from build123d import *

# Parameters (mm, degrees)
BOSS_EXTRUDE1_DEPTH = 30
SKETCH4_W           = 30
SKETCH4_H           = 11.480502971
BOSS_EXTRUDE2_DEPTH = 50
CUT_EXTRUDE1_DEPTH  = 5
CUT_EXTRUDE3_DEPTH  = 6.480502971
FILLET1_R           = 10
CHAMFER3_SIZE       = 22.5
CHAMFER3_SIZE2      = 8.610377228
CHAMFER1_SIZE       = 15
CHAMFER1_SIZE2      = 20.645728807
CHAMFER2_SIZE2      = 20.645728807
CHAMFER2_SIZE       = 15
CUT_EXTRUDE4_DEPTH  = 25
CUT_EXTRUDE5_DEPTH  = 25
SKETCH9_W           = 20.645728807
SKETCH9_H           = 30
CUT_EXTRUDE6_DEPTH  = 40
SKETCH10_W          = 10
SKETCH10_H          = 12.413129657
BOSS_EXTRUDE3_DEPTH = 12
SKETCH11_W          = 31
SKETCH11_H          = 30
CUT_EXTRUDE7_DEPTH  = 2
SKETCH12_W          = 25.5
SKETCH12_H          = 20
CUT_EXTRUDE8_DEPTH  = 4
CHAMFER4_SIZE       = 2
CUT_EXTRUDE9_DEPTH  = 30
SKETCH16_W          = 6
SKETCH16_H          = 20
CUT_EXTRUDE10_DEPTH = 30.1
CHAMFER6_SIZE       = 2
BOSS_EXTRUDE4_DEPTH = 25.5
SKETCH18_W          = 2.6
SKETCH18_H          = 4.5
BOSS_EXTRUDE5_DEPTH = 10
CHAMFER7_SIZE       = 1
FILLET2_R           = 5
CHAMFER8_SIZE       = 8


with BuildPart() as part:
    # Sketch1 → Boss-Extrude1 (new body)
    with BuildSketch(Plane.XY):
        Polygon((0, 216.478440058), (-153.073372946, 153.073372946), (-216.478440058, 0), (-244.194826034, 0), (-244.194826034, 11.480502971), (-176.034378888, 176.034378888), (0, 248.950206067), align=None)
    extrude(amount=BOSS_EXTRUDE1_DEPTH)

    # Sketch4 → Boss-Extrude2 (add)
    with BuildSketch(Plane.ZY.offset(244.194826034)):
        with Locations((15, 5.740251485)):
            Rectangle(SKETCH4_W, SKETCH4_H)
    extrude(amount=BOSS_EXTRUDE2_DEPTH)

    # Sketch5 → Cut-Extrude1 (cut)
    with BuildSketch(Plane(origin=(0, 11.480502971, 0), x_dir=(1, 0, 0), z_dir=(0, 1, 0))):
        with BuildLine():
            Line((-281.694826034, -6), (-256.694826034, -6))
            ThreePointArc((-256.694826034, -6), (-247.694826034, -15), (-256.694826034, -24))
            Line((-256.694826034, -24), (-281.694826034, -24))
            ThreePointArc((-281.694826034, -24), (-290.694826034, -15), (-281.694826034, -6))
        make_face()
    extrude(amount=-CUT_EXTRUDE1_DEPTH, mode=Mode.SUBTRACT)

    # Sketch7 → Cut-Extrude3 (cut)
    with BuildSketch(Plane(origin=(0, 6.480502971, 0), x_dir=(1, 0, 0), z_dir=(0, 1, 0))):
        with BuildLine():
            Line((-256.694826034, -11.5), (-281.694826034, -11.5))
            ThreePointArc((-281.694826034, -11.5), (-285.194826034, -15), (-281.694826034, -18.5))
            Line((-281.694826034, -18.5), (-256.694826034, -18.5))
            ThreePointArc((-256.694826034, -18.5), (-253.194826034, -15), (-256.694826034, -11.5))
        make_face()
    extrude(amount=-CUT_EXTRUDE3_DEPTH, mode=Mode.SUBTRACT)

    # Fillet1
    fillet1_edges = [part.edges().sort_by_distance(p)[0] for p in [
        (-294.194826034, 5.740251485, 0),
        (-294.194826034, 5.740251485, 30),
    ]]
    fillet(fillet1_edges, radius=FILLET1_R)

    # Chamfer3
    chamfer3_edges = [part.edges().sort_by_distance(p)[0] for p in [
        (0, 248.950206067, 15),
    ]]
    chamfer3_side = [part.faces().sort_by_distance(p)[0] for p in [
        (-88.017189444, 212.492292478, 15),
    ]]
    chamfer(chamfer3_edges, length=CHAMFER3_SIZE, length2=CHAMFER3_SIZE2, reference=chamfer3_side[0])

    # Chamfer1
    chamfer1_edges = [part.edges().sort_by_distance(p)[0] for p in [
        (0, 228.409134449, 0),
    ]]
    chamfer1_side = [part.faces().sort_by_distance(p)[0] for p in [
        (0, 228.409134449, 15),
    ]]
    chamfer(chamfer1_edges, length=CHAMFER1_SIZE, length2=CHAMFER1_SIZE2, reference=chamfer1_side[0])

    # Chamfer2
    chamfer2_edges = [part.edges().sort_by_distance(p)[0] for p in [
        (0, 228.409134449, 30),
    ]]
    chamfer2_side = [part.faces().sort_by_distance(p)[0] for p in [
        (0, 228.409134449, 29.7),
    ]]
    chamfer(chamfer2_edges, length=CHAMFER2_SIZE - 0.0001, length2=CHAMFER2_SIZE2 - 0.0001, reference=chamfer2_side[0])  # a hair under: the kernel refuses the full size

    # Sketch3 → Cut-Extrude4 (cut)
    with BuildSketch(Plane.XY.offset(30)):
        Polygon((-186.689323664, 71.91728881), (-182.86248934, 81.156084136), (-192.101284666, 84.982918459), (-184.129988769, 104.227329121), (-202.60757942, 111.880997769), (-206.434413743, 102.642202444), (-194.423979821, 97.667317823), (-203.608382197, 75.494209043), (-197.14122547, 72.815425016), (-195.928118989, 75.744123134), align=None)
        Polygon((-81.156084136, 182.86248934), (-71.91728881, 186.689323664), (-75.744123134, 195.928118989), (-72.815425016, 197.14122547), (-75.494209043, 203.608382197), (-97.667317823, 194.423979821), (-102.642202444, 206.434413743), (-111.880997769, 202.60757942), (-106.906113148, 190.597145497), (-104.227329121, 184.129988769), (-84.982918459, 192.101284666), align=None)
    extrude(amount=-CUT_EXTRUDE4_DEPTH, mode=Mode.SUBTRACT)

    # Sketch8 → Cut-Extrude5 (cut)
    with BuildSketch(Plane.XY.offset(30)):
        Polygon((-66.282610192, 194.435244969), (-67.813343921, 198.130763099), (-66.889464389, 198.513446531), (-70.716298712, 207.752241857), (-71.640178245, 207.369558424), (-73.170911974, 211.065076554), (-72.247032442, 211.447759987), (-74.925816468, 217.914916714), (-46.28555096, 229.778103118), (-43.606766934, 223.31094639), (-38.987369271, 225.224363552), (-37.456635542, 221.528845422), (-42.076033204, 219.61542826), (-38.249198881, 210.376632935), (-33.629801218, 212.290050097), (-32.099067489, 208.594531967), align=None)
    extrude(amount=-CUT_EXTRUDE5_DEPTH, mode=Mode.SUBTRACT)

    # Sketch9 → Cut-Extrude6 (cut)
    with BuildSketch(Plane(origin=(0, 240.339828839, 0), x_dir=(1, 0, 0), z_dir=(0, 1, 0))):
        with Locations((-10.322864404, -15)):
            Rectangle(SKETCH9_W, SKETCH9_H)
    extrude(amount=-CUT_EXTRUDE6_DEPTH, mode=Mode.SUBTRACT)


with BuildPart() as cut_extrude6_kept_piece:
    # of the separate pieces the step leaves, the one the design keeps (cut_extrude6_pieces_kept)
    add(part.part.solids().sort_by_distance((-20.787289482, 240.339828839, 30))[0])

    # Sketch10 → Boss-Extrude3 (add)
    with BuildSketch(Plane(origin=(-20.645728807, 0, 0), x_dir=(0, 0, -1), z_dir=(1, 0, 0))):
        with Locations((-15, 224.13326401)):
            Rectangle(SKETCH10_W, SKETCH10_H)
    extrude(amount=BOSS_EXTRUDE3_DEPTH)

    # Sketch11 → Cut-Extrude7 (cut)
    with BuildSketch(Plane(origin=(-76.536686473, 184.775906502, 0), x_dir=(0.9238795325112865, 0.38268343236509045, 0), z_dir=(0.38268343236509045, -0.9238795325112865, 0))):
        with Locations((0.5, 15)):
            Rectangle(SKETCH11_W, SKETCH11_H)
    extrude(amount=-CUT_EXTRUDE7_DEPTH, mode=Mode.SUBTRACT)

    # Sketch12 → Cut-Extrude8 (cut)
    with BuildSketch(Plane(origin=(-184.775906502, 76.536686473, 0), x_dir=(0, 0, -1), z_dir=(0.9238795325112872, -0.38268343236508917, 0))):
        with Locations((-17.25, 0)):
            Rectangle(SKETCH12_W, SKETCH12_H)
    extrude(amount=-CUT_EXTRUDE8_DEPTH, mode=Mode.SUBTRACT)

    # Chamfer4
    chamfer4_edges = [cut_extrude6_kept_piece.edges().sort_by_distance(p)[0] for p in [
        (-111.880997769, 202.60757942, 17.5),
        (-102.642202444, 206.434413743, 17.5),
        (-83.45218473, 188.405766535, 30),
        (-74.279774075, 196.534672229, 30),
        (-74.154817029, 200.374803834, 30),
        (-86.580763433, 199.016181009, 30),
        (-100.154760133, 200.429196782, 30),
        (-108.054163445, 193.368784094, 30),
        (-94.60512379, 188.115636717, 30),
        (-206.434413743, 102.642202444, 17.5),
        (-188.115636717, 94.60512379, 30),
        (-193.368784094, 108.054163445, 30),
        (-200.429196782, 100.154760133, 30),
        (-199.016181009, 86.580763433, 30),
        (-200.374803834, 74.154817029, 30),
        (-196.534672229, 74.279774075, 30),
        (-193.156480392, 74.596072837, 30),
        (-49.19083884, 201.514888468, 30),
        (-32.864434353, 210.442291032, 30),
        (-40.162616043, 214.996030597, 30),
        (-38.222002407, 223.376604487, 30),
        (-72.40554511, 209.217317489, 30),
        (-67.047977056, 196.283004034, 30),
        (-74.213389405, 192.232600859, 30),
        (-81.921451, 184.710248405, 17.5),
        (-72.682655675, 188.537082729, 17.5),
        (-189.329646068, 83.834868162, 30),
        (-186.55800747, 82.686817865, 17.5),
        (-190.384841794, 73.44802254, 17.5),
    ]]
    chamfer(chamfer4_edges, length=CHAMFER4_SIZE)

    # Sketch13 → Cut-Extrude9 (cut)
    with BuildSketch(Plane(origin=(0, 0, 0), x_dir=(-1, 0, 0), z_dir=(0, 0, -1))):
        Polygon((180.789758921, 164.553875917), (153.073372946, 153.073372946), (-25.433862624, 226.424491684), (-10.416597064, 262.970499532), (187.527299345, 181.632585119), align=None)
    extrude(amount=-CUT_EXTRUDE9_DEPTH, mode=Mode.SUBTRACT)

    # Sketch16 → Cut-Extrude10 (cut)
    with BuildSketch(Plane(origin=(31.702533556, 76.536686473, 0), x_dir=(0.9238795325112868, -0.38268343236508956, 0), z_dir=(0.38268343236508956, 0.9238795325112868, 0))):
        with Locations((-227, -15)):
            Rectangle(SKETCH16_W, SKETCH16_H)
        with Locations((-203, -15)):
            Rectangle(SKETCH16_W, SKETCH16_H)
    extrude(amount=-CUT_EXTRUDE10_DEPTH, mode=Mode.SUBTRACT)

    # Chamfer6
    chamfer6_edges = [cut_extrude6_kept_piece.edges().sort_by_distance(p)[0] for p in [
        (-178.018120324, 163.40582562, 25),
        (-175.246481726, 162.257775323, 15),
        (-178.018120324, 163.40582562, 5),
        (-155.845011544, 154.221423243, 5),
        (-158.616650141, 155.36947354, 15),
        (-155.845011544, 154.221423243, 25),
    ]]
    chamfer(chamfer6_edges, length=CHAMFER6_SIZE)

    # Sketch17 → Boss-Extrude4 (add)
    with BuildSketch(Plane.XY.offset(4.5)):
        Polygon((-188.602740826, 67.297891148), (-191.00482761, 68.292868072), (-189.091410449, 72.912265735), (-186.689323664, 71.91728881), align=None)
        Polygon((-183.351158963, 86.770458722), (-180.949072179, 85.775481798), (-182.86248934, 81.156084136), (-185.264576125, 82.15106106), align=None)
    extrude(amount=BOSS_EXTRUDE4_DEPTH)

    # Sketch18 → Boss-Extrude5 (add)
    with BuildSketch(Plane(origin=(-1.913417162, -4.619397663, 0), x_dir=(0.9238795325112867, -0.38268343236508984, 0), z_dir=(0.38268343236508984, 0.9238795325112867, 0))):
        with Locations((-201.3, -27.75)):
            Rectangle(SKETCH18_W, SKETCH18_H)
    extrude(amount=BOSS_EXTRUDE5_DEPTH)

    # Chamfer7
    chamfer7_edges = [cut_extrude6_kept_piece.edges().sort_by_distance(p)[0] for p in [
        (-185.218615457, 85.920396229, 30),
        (-191.724233807, 70.214444176, 30),
        (-187.177993287, 77.531663397, 30),
    ]]
    chamfer(chamfer7_edges, length=CHAMFER7_SIZE)

    # Fillet2
    fillet2_edges = [cut_extrude6_kept_piece.edges().sort_by_distance(p)[0] for p in [
        (-187.890367056, 72.414777273, 25.5),
        (-184.063532733, 81.653572598, 25.5),
        (-184.063532733, 81.653572598, 4.5),
        (-187.890367056, 72.414777273, 4.5),
    ]]
    fillet(fillet2_edges, radius=FILLET2_R - 0.0001)  # a hair under: the kernel refuses the full size

    # Chamfer8
    chamfer8_edges = [cut_extrude6_kept_piece.edges().sort_by_distance(p)[0] for p in [
        (-202.60757942, 111.880997769, 16.5),
    ]]
    chamfer(chamfer8_edges, length=CHAMFER8_SIZE)


solid = cut_extrude6_kept_piece.part
Design review of the part built by this model. Coordinates are the model's own, in mm. A direction names the side the tool comes from. Coordinates: 2 decimals unless noted, no trailing zeros. Loops run counter-clockwise (first coordinate to the right, second up) from the corner with the lowest first, then second, coordinate; pieces in that order, holes last. Notation, with made-up numbers: (-4, 44) -> (16, 44) arc R33 cw to (16, 83) -> close; hole circle Ø10 at (-25.5, -7). An arc over 180 degrees is marked (long way). Use a Markdown table: item, result. Add a question column.
Item 1: The part is to be moulded in two halves that separate along X. For faces 1 (the flat face through (-204, 76, 0)), 2 (the cylindrical face through (-187.33, 73.73, 24)), 3 (the flat face through (-191.288, 71.267, 17.715)), say which applies: +X half, -X half, draft (parallel to the pull), parting line (faces both ways), or undercut.
Item 2: We need section A-A, the plane x = -274. Write out the cut boundary in (y, z), and give its area (3 significant figures).
Item 3: We need section D-D, the plane x = -210.5. Write out the cut boundary in (y, z), and give its area (3 significant figures).
Item 4: We need section B-B, the plane z = 15. Count the separate pieces of the cut face and the enclosed holes in it, and give its area (3 significant figures).
Item 5: Clearance check with flat-ended pins moving along their axes: P1, Ø1.5, axis at y = 80.5, z = 23, coming from the -X side; P2, Ø14.5, axis at x = -279.5, z = 12.5, coming from the +Y side; P3, Ø12, axis at x = -189.5, y = 42.5, coming from the +Z side (3 decimals); P4, Ø3, axis at x = -192.5, z = 8, coming from the -Y side. State where each tip first meets the part, or that it passes through.
Item 6: We need section C-C, the plane y = 131.5. Write out the cut boundary in (x, z).
Item 7: Wall thickness on L1, parallel to Y at x = -187, z = 17.5; L2, parallel to Y at x = -197, z = 17.5; L3, parallel to X at y = 86.5, z = 20.5: over which ranges is each line inside the solid? List them lowest first. Write a range as from..to.
Item 8: Machinability: for faces 4 (the flat face through (-164.683, 140.723, 15.14)), 5 (the flat face through (-188.17, 94.47, 16.66)), 6 (the flat face through (-189.192, 107.392, 28.986)), 7 (the cylindrical face through (-253.196, 3.286, 15.077)), 8 (the flat face through (-178.355, 162.448, 25.986)), which of the approach directions +Z, -Z, +X, -X, +Y, -Y give a long, thin tool a straight path to every point of the face, cutting with its end or side? Answer none if there is none.
Numbers:
| question | item | result |
|---|---|---|
| 1 | face 1 | draft |
| 1 | face 2 | +X half |
| 1 | face 3 | undercut |
| 2 | outline | (0, 0) -> (11.48, 0) -> (11.48, 6) -> (6.48, 6) -> (6.48, 11.5) -> (0, 11.5) -> close; (0, 18.5) -> (6.48, 18.5) -> (6.48, 24) -> (11.48, 24) -> (11.48, 30) -> (0, 30) -> close |
| 2 | area | 209 mm^2 |
| 3 | outline | (14.43, 0) -> (92.83, 0) -> (92.83, 30) -> (14.43, 30) -> close |
| 3 | area | 2,350 mm^2 |
| 4 | separate pieces | 3 |
| 4 | enclosed holes | 0 |
| 4 | area | 4,400 mm^2 |
| 5 | P1 | stops at x = -215.92 |
| 5 | P2 | stops at y = 11.48 |
| 5 | P3 | passes through |
| 5 | P4 | stops at y = 54.27 |
| 6 | outline | (-194.48, 0) -> (-162.01, 0) -> (-162.01, 5) -> (-168.5, 5) -> (-168.5, 25) -> (-162.01, 25) -> (-162.01, 30) -> (-194.48, 30) -> close |
| 7 | L1 | y = 71.17..72.05, 84.03..97.3, 105.42..134.55 |
| 7 | L2 | y = 47.03..73.16, 91.45..98.73, 113.13..125.42 |
| 7 | L3 | x = -213.12..-199.05, -191.47..-184.98, -183.46..-180.65 |
| 8 | face 4 | +X |
| 8 | face 5 | +Z |
| 8 | face 6 | +Z, -X |
| 8 | face 7 | +Y, -Y |
| 8 | face 8 | +Y |
